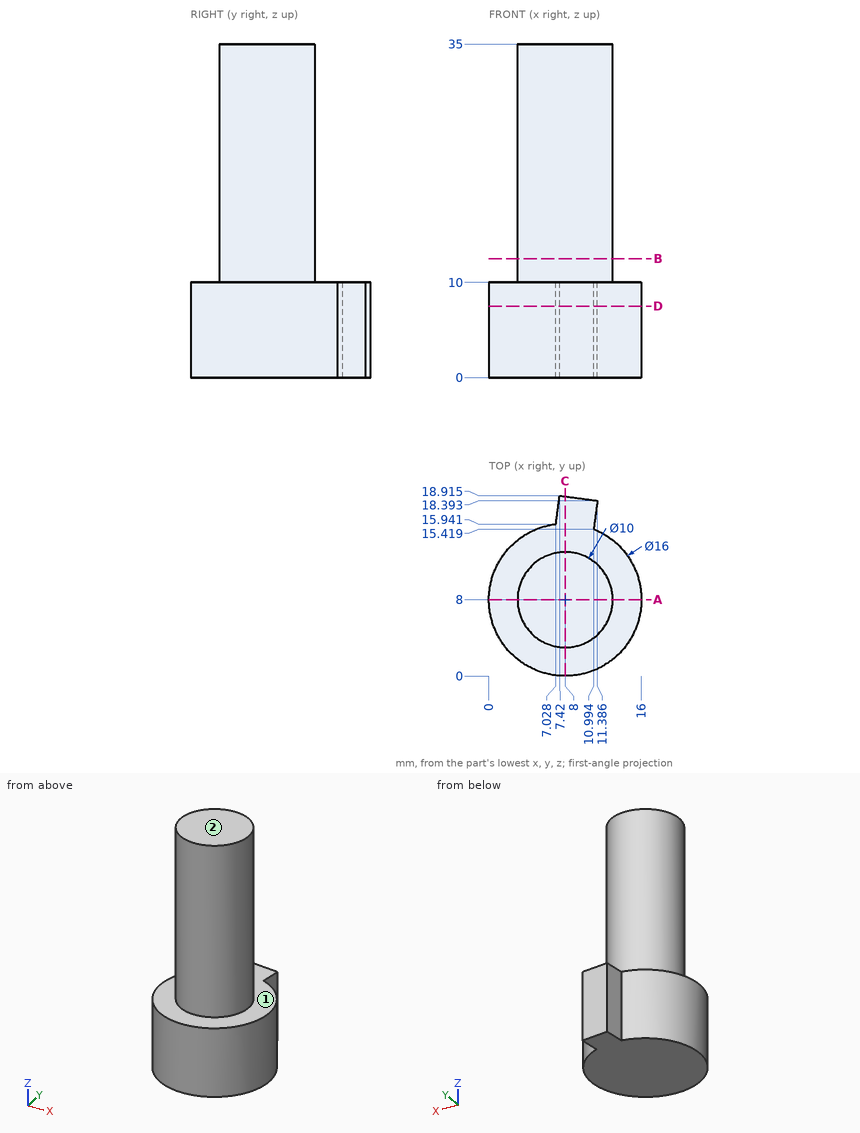
Geometry: see drawing. Coordinates: mm, zero at the bounding-box minimum. A direction names the side the tool comes from. Round coordinates to 2 decimals unless told otherwise and drop trailing zeros. Write each loop counter-clockwise with the first axis right and the second up, starting at its lowest first coordinate (ties: lowest second). Pieces come first, ordered by that corner, then holes. Notation, with made-up numbers: M -40,65 L 0,65 A10 cw 0,73 Z; hole C -35.75,3.5 d8. An arc over 180 degrees is marked long. Answer in a Markdown table with one row per item. Add a question column.
(1) Cut plane A-A, the plane y = 8. Return the cut outline in (x, z), then the cut area to 3 significant figures.
(2) Ray query, L1, parallel to Z at x = 9, y = 15; L2, parallel to X at y = 15, z = 7 (1 decimal); L3, parallel to X at y = 5.5, z = 26.5. Return the intervals inside material, ascending.
(3) Cut plane B-B, the plane z = 12.5. Return the cut outline in (x, y).
(4) Reachability of the marked faces 1 and 2 from +Z, -Z, +X, -X, +Y, -Y: full face, straight path, thin tool, end or side. Return the list, or none.
(5) Contact query for flat-ended pins moving along their axis: pin 1 (8 mm diameter, centred on y = 2.5, z = 13.5, fed in from +X); pin 2 (1 mm diameter, centred on y = 3.5, z = 30, fed in from +X); pin 3 (4 mm diameter, centred on y = 15.5, z = 5, fed in from +X). Output: stop coordinate, or through.
(6) Cut plane C-C, the plane x = 8. Return the cut outline in (y, z), then the cut area to 3 significant figures.
(7) Cut plane D-D, the plane z = 7.5. Return the cut outline in (x, y) (1 decimal), then the cut area to 3 significant figures.
Established:
| question | item | result |
|---|---|---|
| 1 | outline | M 0,0 L 16,0 L 16,10 L 13,10 L 13,35 L 3,35 L 3,10 L 0,10 Z |
| 1 | area | 410 mm² |
| 2 | L1 | 0 to 10 |
| 2 | L2 | 4.1 to 11.9 |
| 2 | L3 | 3.67 to 12.33 |
| 3 | outline | C 8,8 d10 |
| 4 | face 1 | +Z |
| 4 | face 2 | +Z, +X, -X, +Y, -Y |
| 5 | pin 1 | x = 15.16 |
| 5 | pin 2 | x = 11 |
| 5 | pin 3 | x = 13.81 |
| 6 | outline | M 0,0 L 18.84,0 L 18.84,10 L 13,10 L 13,35 L 3,35 L 3,10 L 0,10 Z |
| 6 | area | 438 mm² |
| 7 | outline | M 7,15.9 A8 ccw long 11,15.4 L 11.4,18.4 L 7.4,18.9 Z |
| 7 | area | 212 mm² |
